Read the model definition and answer for the solid it produces. Units are mm, in the model's axes. Give positions to 0.01 mm unless a question says otherwise; leave off trailing zeros. Order: outer loops, then holes, each group sorted by start corner. A loop starts at its lowest first (then second) coordinate and runs counter-clockwise, first axis right, second up. Notation, with made-up numbers: (-14.5, 12.5) -> (12.5, 12.5) arc R7 ccw to (12.5, 16.5) -> close; hole circle Ø6 at (-1, 33.25). An arc over 180 degrees is marked (long way). Use one line per item in the form item = value.
```python
from build123d import *

# Parameters (mm, degrees)
SKETCH1_W               = 552.45
SKETCH1_H               = 19.05
BOSS_EXTRUDE1_DEPTH     = 6.35
CUT_EXTRUDE1_DEPTH      = 277.680802099
CUT_EXTRUDE1_DEPTH_BACK = 277.680802099
SKETCH2_R               = 5.588
FILLET1_R               = 2.54


with BuildPart() as part:
    # Sketch1 → Boss-Extrude1 (new, symmetric)
    with BuildSketch(Plane.XY):
        Rectangle(SKETCH1_W, SKETCH1_H)
    extrude(amount=BOSS_EXTRUDE1_DEPTH, both=True)

    # Sketch2 → Cut-Extrude1 (cut, two sides: drawn at the far end of the back side and taken through both)
    with BuildSketch(Plane.XY.offset(6.35).offset(-CUT_EXTRUDE1_DEPTH_BACK)):
        Circle(SKETCH2_R)
        with Locations((-250.825, 0)):
            Circle(SKETCH2_R)
    extrude(amount=CUT_EXTRUDE1_DEPTH + CUT_EXTRUDE1_DEPTH_BACK, mode=Mode.SUBTRACT)

    # Fillet1
    fillet1_edges = [part.edges().sort_by_distance(p)[0] for p in [
        (-276.225, 0, 6.35),
        (276.225, 0, 6.35),
        (-276.225, 0, -6.35),
        (276.225, 0, -6.35),
    ]]
    fillet(fillet1_edges, radius=FILLET1_R)


solid = part.part
```
Item 1: The part is cut by section A-A on x = 0. Give the vertices of the cut face in (y, z) (3 decimals), and give its area (4 significant figures).
Checks:
outline = (-9.525, -6.35) -> (-5.588, -6.35) -> (-5.588, 6.35) -> (-9.525, 6.35) -> close; (5.588, -6.35) -> (9.525, -6.35) -> (9.525, 6.35) -> (5.588, 6.35) -> close
area = 100.0 mm²
Item 2: Given pin 1 Ø6.5 at (x, y) = (-250.825, 0) entering from +Z, flat-ended and moving along its own axis, determine where the tip first touches the part or whether it passes through.
Checks:
pin_1 = through
Item 3: Determine the mould class of faces 1 (the flat face through (-4, 9.525, 0)), 2 (the flat face through (-4, -9.525, 0)), 3 (the cylindrical face through (-4.434, -3.4, -0.089)) for opening direction Y: +Y half, -Y half, draft (parallel to the pull), parting line (faces both ways), or undercut.
Checks:
face_1 = +Y half
face_2 = -Y half
face_3 = undercut
Item 4: The part is cut by section B-B on y = 0. Give the vertices of the cut face in (x, z) (3 decimals), and give its area (3 significant figures).
Checks:
outline = (-276.225, -3.81) arc R2.54 ccw to (-273.685, -6.35) -> (-256.413, -6.35) -> (-256.413, 6.35) -> (-273.685, 6.35) arc R2.54 ccw to (-276.225, 3.81) -> close; (-245.237, -6.35) -> (-5.588, -6.35) -> (-5.588, 6.35) -> (-245.237, 6.35) -> close; (5.588, -6.35) -> (273.685, -6.35) arc R2.54 ccw to (276.225, -3.81) -> (276.225, 3.81) arc R2.54 ccw to (273.685, 6.35) -> (5.588, 6.35) -> close
area = 6,730 mm²
Item 5: Straight lines are drawn through the part: L1, parallel to X at y = 0, z = -3 (3 decimals); L2, parallel to Y at x = 0, z = 1.25 (3 decimals); L3, parallel to X at y = -3.25, z = -1.5 (3 decimals). For each, find the intervals that lie inside material, in ascending order. Write a range as from..to.
Checks:
L1 = -276.225..-256.413, -245.237..-5.588, 5.588..276.225
L2 = -9.525..-5.588, 5.588..9.525
L3 = -276.225..-255.371, -246.279..-4.546, 4.546..276.225
